from build123d import *

# Parameters (mm, degrees)
CUT_EXTRUDE_START   = 6.5
CUT_EXTRUDE_1_DEPTH = 95.495049384


with BuildPart() as part:
    # Эскиз1 → Повернуть1 (revolve)
    with BuildSketch(Plane.XY, mode=Mode.PRIVATE) as revolve_1_sk:
        Polygon((0, 0), (0, 8.5), (12, 8.5), (12, 10), (67, 10), (67, 8.5), (79, 8.5), (79, 8), (100, 8), (100, 0), align=None)
    revolve(revolve_1_sk.sketch.rotate(Axis((100, 0, 0), (-1, 0, 0)), 90), axis=Axis((100, 0, 0), (-1, 0, 0)))

    # Эскиз2 → Вырез-Вытянуть1 (cut, through all)
    with BuildSketch(Plane(origin=(0, 0, 0), x_dir=(1, 0, 0), z_dir=(0, 1, 0)).offset(CUT_EXTRUDE_START)):
        with BuildLine():
            Line((28.5, 3), (50.5, 3))
            ThreePointArc((50.5, 3), (53.5, 0), (50.5, -3))
            Line((50.5, -3), (28.5, -3))
            ThreePointArc((28.5, -3), (25.5, 0), (28.5, 3))
        make_face()
    extrude(amount=CUT_EXTRUDE_1_DEPTH, mode=Mode.SUBTRACT)


solid = part.part
Read the model definition and answer for the solid it produces. Units are mm, in the model's axes. A direction names the side the tool comes from. Round coordinates to 2 decimals unless told otherwise and drop trailing zeros. Order: outer loops, then holes, each group sorted by start corner. A loop starts at its lowest first (then second) coordinate and runs counter-clockwise, first axis right, second up.
1) The part is cut by section B-B on z = 0. Write down the section's boundary in (x, y), plus the area to 3 significant figures.
2) For faces 1 (the face through (100, 0, 0)), 2 (the face through (53.5, 8.2, -0.1)), 3 (the face through (89.65, 7.81, 1.73)), determine the directions among +Z, -Z, +X, -X, +Y, -Y from which every point of the face is accessible in a straight line to the end or side of a thin tool.
3) Flat-ended cylindrical pins translate along their axes: pin 1 (1.5 mm diameter, centred on x = 39, y = 7.5, fed in from -Z); pin 2 (3 mm diameter, centred on x = 39.5, z = 0.5, fed in from +Y); pin 3 (8 mm diameter, centred on x = 86.5, z = 3.5, fed in from -Y). Find the tip coordinate at first contact, or state that the pin passes through.
4) The part is cut by section D-D on y = -5.5. Write down the section's boundary in (x, z).
5) The mould has two halves that part along X. Classify faces 4 (the face through (40, 6.5, 0)), 5 (the face through (6.084, -8.428, 1.107)), 6 (the face through (12, 7.4, -4.5)): released by +X, released by -X, zero draft, split by the parting line, or undercut.
6) The part is cut by section A-A on y = 0. Write down the section's boundary in (x, z).
7) The part is cut by section C-C on x = 10. Write down the section's boundary in (y, z), plus the area to 3 significant figures.
8) Straight lines are drawn through the part: L1, parallel to Z at x = 89.5, y = 0.5; L2, parallel to Y at x = 69, z = 0; L3, parallel to Y at x = 4, z = 4.5. For each, find the intervals that lie inside material, in ascending order.
Resolved:
1. outline: (0, -8.5) - (12, -8.5) - (12, -10) - (67, -10) - (67, -8.5) - (79, -8.5) - (79, -8) - (100, -8) - (100, 8) - (79, 8) - (79, 8.5) - (67, 8.5) - (67, 10) - (53.5, 10) - (53.5, 6.5) - (25.5, 6.5) - (25.5, 10) - (12, 10) - (12, 8.5) - (0, 8.5) - close
1. area: 1,750 mm2
2. face 1: +Z, -Z, +X, +Y, -Y
2. face 2: +Y
2. face 3: +X
3. pin 1: stops at z = -7.38
3. pin 2: stops at y = 6.5
3. pin 3: stops at y = -8
4. outline: (0, -6.48) - (12, -6.48) - (12, -8.35) - (67, -8.35) - (67, -6.48) - (79, -6.48) - (79, -5.81) - (100, -5.81) - (100, 5.81) - (79, 5.81) - (79, 6.48) - (67, 6.48) - (67, 8.35) - (12, 8.35) - (12, 6.48) - (0, 6.48) - close
5. face 4: undercut
5. face 5: zero draft
5. face 6: released by -X
6. outline: (0, -8.5) - (12, -8.5) - (12, -10) - (67, -10) - (67, -8.5) - (79, -8.5) - (79, -8) - (100, -8) - (100, 8) - (79, 8) - (79, 8.5) - (67, 8.5) - (67, 10) - (12, 10) - (12, 8.5) - (0, 8.5) - close
7. outline: circle Ø17 at (0, 0)
7. area: 227 mm2
8. L1: z = -7.98 to 7.98
8. L2: y = -8.5 to 8.5
8. L3: y = -7.21 to 7.21
